Work out the finished part from the listing and answer in its coordinate system (mm). Round coordinates to 2 decimals unless told otherwise and drop trailing zeros. Write each loop counter-clockwise with the first axis right and the second up, starting at its lowest first coordinate (ties: lowest second). Pieces come first, ordered by that corner, then holes. Notation, with made-up numbers: (-13, -34.75) -> (6, -34.75) arc R15 cw to (6, -18.75) -> close; hole circle Ø1 at (-38, -7). An arc over 180 degrees is marked (long way). Answer as a JSON object with one key per item and string values. Group by question number.
Autodesk Inventor part; units mm, degrees
ref_plane "YZ Plane" through (0, 0, 0) normal (1, 0, 0) x (0, 1, 0)
ref_plane "XZ Plane" through (0, 0, 0) normal (0, 1, 0) x (-1, 0, 0)
ref_plane "XY Plane" through (0, 0, 0) normal (0, 0, 1) x (1, 0, 0)
sketch "Szkic1" plane through (0, 0, 0) normal (0, 0, 1) x (1, 0, 0)
  line L0 (-16.0262, 157.75) -> (-18.2115, 157.75)
  line L1 (-18, 155.6545) -> (-18, 158.2708)
  line L2 (-16, 157.75) -> (18, 157.75)
  line L3 (18, 157.75) -> (17.9772, 121.6933)
  line L4 (17.9772, 121.6933) -> (-18.0451, 121.7161)
  line L5 (-18.0451, 121.7161) -> (-18, 157.75)
  circle A0 centre (-14.4, 154.15) radius 2
  circle A1 centre (14.4, 154.15) radius 2
  circle A2 centre (14.4, 125.35) radius 2
  circle A3 centre (-14.4, 125.35) radius 2
  line L6 (17.9772, 121.6933) -> (-18, 121.6933)
  line L7 (-18, 121.6933) -> (-18, 157.75)
  line L8 (-18, 157.75) -> (17.9772, 157.75)
  line L9 (17.9772, 157.75) -> (17.9772, 121.6933)
  circle A4 centre (-14.4, 154.15) radius 2
  circle A5 centre (14.4, 154.15) radius 2
  circle A6 centre (14.4, 125.35) radius 2
  circle A7 centre (-14.4, 125.35) radius 2
  point P0 (0, 0)
  point P1 (17.9772, 157.75)
  point P2 (-18, 121.7161)
extrude "Wyciągnięcie proste1" add sketch "Szkic1" along normal blind 1.5 contours L8 L2 L9 L4 L7 L1 L0
properties part number "płytka"
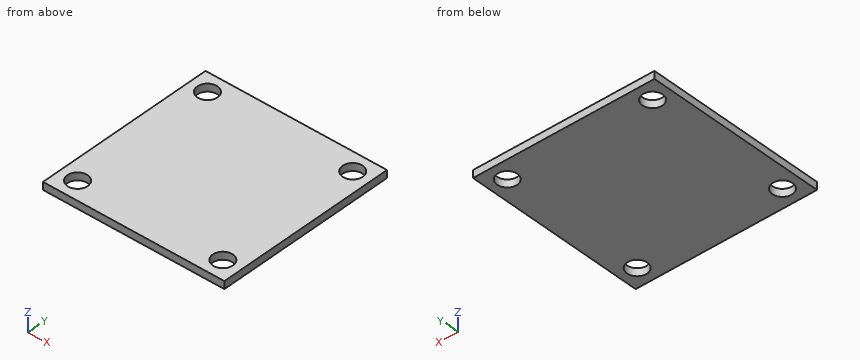
1) A cutting plane is placed at C-C on x = 14. Determine the outline of the cut face in (y, z), plus the area to 3 significant figures.
2) A cutting plane is placed at A-A on y = 154.15. Determine the outline of the cut face in (x, z).
3) Straight lines are drawn through the part: L1, parallel to Y at x = -14.4, z = 0.4; L2, parallel to X at y = 125.5, z = 1.2; L3, parallel to X at y = 153.5, z = 1.4. For each, find the intervals that lie inside material, in ascending order.
4) A cutting plane is placed at B-B on z = 1. Determine the outline of the cut face in (x, y).
5) This flat-tipped pin is pushed along its axis until it touches: P1, Ø3.5, axis at x = -14.4, y = 125.35, coming from the -Z side. Where does it stop, or does it pass through?
Established:
{
 "1": {"outline": "(121.7, 0) -> (123.39, 0) -> (123.39, 1.5) -> (121.7, 1.5) -> close; (127.31, 0) -> (152.19, 0) -> (152.19, 1.5) -> (127.31, 1.5) -> close; (156.11, 0) -> (157.75, 0) -> (157.75, 1.5) -> (156.11, 1.5) -> close", "area": "42.3 mm²"},
 "2": {"outline": "(-18, 0) -> (-16.4, 0) -> (-16.4, 1.5) -> (-18, 1.5) -> close; (-12.4, 0) -> (12.4, 0) -> (12.4, 1.5) -> (-12.4, 1.5) -> close; (16.4, 0) -> (17.98, 0) -> (17.98, 1.5) -> (16.4, 1.5) -> close"},
 "3": {"L1": "y = 121.71 to 123.35, 127.35 to 152.15, 156.15 to 157.75", "L2": "x = -18 to -16.39, -12.41 to 12.41, 16.39 to 17.98", "L3": "x = -18 to -16.29, -12.51 to 12.51, 16.29 to 17.98"},
 "4": {"outline": "(-18, 121.72) -> (17.98, 121.69) -> (17.98, 157.75) -> (-18, 157.75) -> close; hole circle Ø4 at (-14.4, 125.35); hole circle Ø4 at (-14.4, 154.15); hole circle Ø4 at (14.4, 125.35); hole circle Ø4 at (14.4, 154.15)"},
 "5": {"P1": "passes through"}
}
